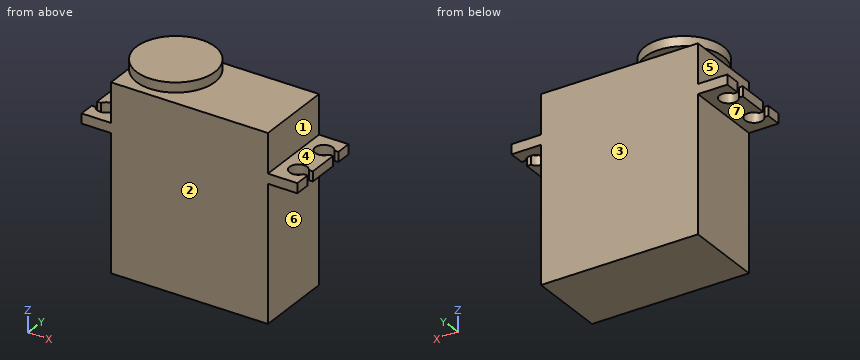
```python
from build123d import *

# Parameters (mm, degrees)
SKETCH1_W           = 47
SKETCH1_H           = 20
BOSS_EXTRUDE1_DEPTH = 40
SKETCH2_R           = 2.95
BOSS_EXTRUDE5_DEPTH = 4
SKETCH5_R           = 10
BOSS_EXTRUDE6_DEPTH = 2.5
SKETCH6_W           = 2.5
SKETCH6_H           = 20
BOSS_EXTRUDE7_DEPTH = 7.5
CUT_EXTRUDE1_REACH  = 60.043
SKETCH7_R           = 2.25


with BuildPart() as part:
    # Sketch1 → Boss-Extrude1 (new body)
    with BuildSketch(Plane(origin=(0, 0, 0), x_dir=(0, 0, -1), z_dir=(1, 0, 0))):
        with Locations((23.5, 10)):
            Rectangle(SKETCH1_W, SKETCH1_H)
    extrude(amount=BOSS_EXTRUDE1_DEPTH)

    # Sketch2 → Boss-Extrude5 (add)
    with BuildSketch(Plane.XY):
        with Locations(Location((10, 10, 0), (0, 0, 180))):
            Circle(SKETCH2_R)
    extrude(amount=BOSS_EXTRUDE5_DEPTH)

    # Sketch5 → Boss-Extrude6 (add)
    with BuildSketch(Plane.XY.offset(4)):
        with Locations((10, 10)):
            Circle(SKETCH5_R)
    extrude(amount=-BOSS_EXTRUDE6_DEPTH)

    # Sketch6 → Boss-Extrude7 (add)
    with BuildSketch(Plane.ZY):
        with Locations((-11.25, 10)):
            Rectangle(SKETCH6_W, SKETCH6_H)
    boss_extrude7 = extrude(amount=BOSS_EXTRUDE7_DEPTH)

    # Sketch7 → Cut-Extrude1 (cut, up to next)
    with BuildSketch(Plane.XY.offset(-10), mode=Mode.PRIVATE) as cut_extrude1_sk1:
        with Locations((-4.5, 15)):
            Circle(SKETCH7_R)
    cut_extrude1_tool1 = extrude(cut_extrude1_sk1.sketch, amount=-CUT_EXTRUDE1_REACH, mode=Mode.PRIVATE) & part.part
    # Sketch7 → Cut-Extrude1 (cut, up to next)
    with BuildSketch(Plane.XY.offset(-10), mode=Mode.PRIVATE) as cut_extrude1_sk2:
        with BuildLine():
            ThreePointArc((-6.489974874, 13.95), (-6.75, 15), (-6.489974874, 16.05))
            Line((-6.489974874, 16.05), (-7.5, 16.05))
            Line((-7.5, 16.05), (-7.5, 13.95))
            Line((-7.5, 13.95), (-6.489974874, 13.95))
        make_face()
    cut_extrude1_tool2 = extrude(cut_extrude1_sk2.sketch, amount=-CUT_EXTRUDE1_REACH, mode=Mode.PRIVATE) & part.part
    # Sketch7 → Cut-Extrude1 (cut, up to next)
    with BuildSketch(Plane.XY.offset(-10), mode=Mode.PRIVATE) as cut_extrude1_sk3:
        with Locations((-4.5, 5)):
            Circle(SKETCH7_R)
    cut_extrude1_tool3 = extrude(cut_extrude1_sk3.sketch, amount=-CUT_EXTRUDE1_REACH, mode=Mode.PRIVATE) & part.part
    # Sketch7 → Cut-Extrude1 (cut, up to next)
    with BuildSketch(Plane.XY.offset(-10), mode=Mode.PRIVATE) as cut_extrude1_sk4:
        with BuildLine():
            Line((-6.489974874, 6.05), (-7.5, 6.05))
            Line((-7.5, 6.05), (-7.5, 3.95))
            Line((-7.5, 3.95), (-6.489974874, 3.95))
            ThreePointArc((-6.489974874, 3.95), (-6.75, 5), (-6.489974874, 6.05))
        make_face()
    cut_extrude1_tool4 = extrude(cut_extrude1_sk4.sketch, amount=-CUT_EXTRUDE1_REACH, mode=Mode.PRIVATE) & part.part
    cut_extrude1_1 = cut_extrude1_tool1.solids().sort_by_distance((-4.5, 15, -10))[0]
    add(cut_extrude1_1, mode=Mode.SUBTRACT)
    cut_extrude1_2 = cut_extrude1_tool2.solids().sort_by_distance((-7.079182, 15, -10))[0]
    add(cut_extrude1_2, mode=Mode.SUBTRACT)
    cut_extrude1_3 = cut_extrude1_tool3.solids().sort_by_distance((-4.5, 5, -10))[0]
    add(cut_extrude1_3, mode=Mode.SUBTRACT)
    cut_extrude1_4 = cut_extrude1_tool4.solids().sort_by_distance((-7.079182, 5, -10))[0]
    add(cut_extrude1_4, mode=Mode.SUBTRACT)
    cut_extrude1 = cut_extrude1_1 + cut_extrude1_2 + cut_extrude1_3 + cut_extrude1_4  # Cut-Extrude1 as one shape, for the pattern or mirror that repeats it

    # Mirror1: Boss-Extrude7, Cut-Extrude1 across plane
    add(boss_extrude7.mirror(Plane(origin=(20, 0, 0), x_dir=(0, 0, 1), z_dir=(1, 0, 0))))
    add(cut_extrude1.mirror(Plane(origin=(20, 0, 0), x_dir=(0, 0, 1), z_dir=(1, 0, 0))), mode=Mode.SUBTRACT)


solid = part.part
```
The listing builds one solid part. Answer for the finished solid, in the listing's coordinates (mm). Face numbers are marked on the shaded views. A direction names the side the tool comes from. Coordinates: 2 decimals unless noted, no trailing zeros. Loops run counter-clockwise (first coordinate to the right, second up) from the corner with the lowest first, then second, coordinate; pieces in that order, holes last. Notation, with made-up numbers: M 37.25,54.5 L 56.25,54.5 A31 cw 56.25,93.5 Z; hole C 82,38 d9. An arc over 180 degrees is marked long. Answer as a JSON object with one key per item and string values. Group by question number.
Item 1: Section B-B (z = -11) is taken. Write down the section's boundary in (x, y).
Item 2: Section C-C (x = 10) is taken. Write down the section's boundary in (y, z), and give its area (3 significant figures).
Item 3: Each of these flat-tipped pins is pushed along its axis until it touches: P1, Ø6, axis at x = 29.5, y = 3.5, coming from the +Z side; P2, Ø4, axis at x = 45, y = 7.5, coming from the +Z side; P3, Ø10, axis at y = 14.5, z = -38, coming from the -X side. Where does it stop, or does it pass through?
Item 4: Which of the six approach directions +Z, -Z, +X, -X, +Y, -Y give full straight-line access (tool end or side, diameter ignored) to the marked faces 4, 5, 6 and 7?
Item 5: Section D-D (y = 10) is taken. Write down the section's boundary in (x, z).
Item 6: Consider L1, parallel to Y at x = -4.5, z = -11.15; L2, parallel to Z at x = 11.5, y = 7.25; L3, parallel to X at y = 15.5, z = -36.5. Determine where each line is inside the solid, lowest interval first.
Item 7: Section A-A (x = 44.5) is taken. Write down the section's boundary in (y, z).
Item 8: Determine the mould class of the marked faces 1, 2 and 3 for opening direction Y: +Y half, -Y half, draft (parallel to the pull), parting line (faces both ways), or undercut.
Solved:
{
 "1": {"outline": "M -7.5,0 L 47.5,0 L 47.5,3.95 L 46.49,3.95 A2.25 cw long 46.49,6.05 L 47.5,6.05 L 47.5,13.95 L 46.49,13.95 A2.25 cw long 46.49,16.05 L 47.5,16.05 L 47.5,20 L -7.5,20 L -7.5,16.05 L -6.49,16.05 A2.25 cw long -6.49,13.95 L -7.5,13.95 L -7.5,6.05 L -6.49,6.05 A2.25 cw long -6.49,3.95 L -7.5,3.95 Z"},
 "2": {"outline": "M 0,-47 L 20,-47 L 20,0 L 12.95,0 L 12.95,1.5 L 20,1.5 L 20,4 L 0,4 L 0,1.5 L 7.05,1.5 L 7.05,0 L 0,0 Z", "area": "999 mm2"},
 "3": {"P1": "stops at z = 0", "P2": "stops at z = -10", "P3": "stops at x = 0"},
 "4": {"face 4": "+Z, +X, +Y, -Y", "face 5": "+Z, -X, +Y, -Y", "face 6": "-Z, +X, +Y, -Y", "face 7": "-Z, -X, +Y, -Y"},
 "5": {"outline": "M -7.5,-12.5 L 0,-12.5 L 0,-47 L 40,-47 L 40,-12.5 L 47.5,-12.5 L 47.5,-10 L 40,-10 L 40,0 L 12.95,0 L 12.95,1.5 L 20,1.5 L 20,4 L 0,4 L 0,1.5 L 7.05,1.5 L 7.05,0 L 0,0 L 0,-10 L -7.5,-10 Z"},
 "6": {"L1": "y = 0 to 2.75, 7.25 to 12.75, 17.25 to 20", "L2": "z = -47 to 0, 1.5 to 4", "L3": "x = 0 to 40"},
 "7": {"outline": "M 0,-12.5 L 2.75,-12.5 L 2.75,-10 L 0,-10 Z; M 7.25,-12.5 L 12.75,-12.5 L 12.75,-10 L 7.25,-10 Z; M 17.25,-12.5 L 20,-12.5 L 20,-10 L 17.25,-10 Z"},
 "8": {"face 1": "draft", "face 2": "-Y half", "face 3": "+Y half"}
}
